```python
from build123d import *

# Parameters (mm, degrees)
BOSS_EXTRUDE1_DEPTH = 25.4
CUT_EXTRUDE1_DEPTH  = 46.597466007


with BuildPart() as part:
    # Sketch1 → Boss-Extrude1 (new body)
    with BuildSketch(Plane.XY):
        Polygon((-31.75, 15.875), (31.75, 15.875), (13.235753401, -19.110856459), (11.70910986, -20.6375), (-11.70910986, -20.6375), (-13.235753401, -19.110856459), align=None)
    extrude(amount=BOSS_EXTRUDE1_DEPTH)

    # Sketch2 → Cut-Extrude1 (cut, through all)
    with BuildSketch(Plane(origin=(0, 0, 0), x_dir=(-1, 0, 0), z_dir=(0, 0, -1))):
        with BuildLine():
            ThreePointArc((-7.4549, -15.76028553), (-9.525, -13.69018553), (-11.5951, -15.76028553))
            ThreePointArc((-11.5951, -15.76028553), (-9.525, -17.83038553), (-7.4549, -15.76028553))
        make_face()
        with BuildLine():
            ThreePointArc((11.5951, -15.76028553), (9.525, -13.69018553), (7.4549, -15.76028553))
            ThreePointArc((7.4549, -15.76028553), (9.525, -17.83038553), (11.5951, -15.76028553))
        make_face()
        with BuildLine():
            ThreePointArc((17.83038553, 9.525), (15.76028553, 11.5951), (13.69018553, 9.525))
            ThreePointArc((13.69018553, 9.525), (15.76028553, 7.4549), (17.83038553, 9.525))
        make_face()
        with BuildLine():
            ThreePointArc((-13.69018553, 9.525), (-15.76028553, 11.5951), (-17.83038553, 9.525))
            ThreePointArc((-17.83038553, 9.525), (-15.76028553, 7.4549), (-13.69018553, 9.525))
        make_face()
        with BuildLine():
            ThreePointArc((-14.2875, 0), (0, -14.2875), (14.2875, 0))
            ThreePointArc((14.2875, 0), (0, 14.2875), (-14.2875, 0))
        make_face()
    extrude(amount=-CUT_EXTRUDE1_DEPTH, mode=Mode.SUBTRACT)


solid = part.part
```
Could you check a few things on this model? Use its own coordinates, in mm. Round coordinates to 2 decimals unless told otherwise and drop trailing zeros. Loops run counter-clockwise (first coordinate to the right, second up) from the corner with the lowest first, then second, coordinate; pieces in that order, holes last. Notation, with made-up numbers: M 68.5,67 L 123.5,67 A36 ccw 123.5,101 Z; hole C -33,20.25 d9. An arc over 180 degrees is marked long. Put each result on its own line as item: value.
Q1. I need wall thicknesses on probe 1 along Y at (x, z) = (0, 8) (1 decimal); probe 2 along Y at (x, z) = (-9, 12.75) (1 decimal); probe 3 along X at (y, z) = (11, 20.75). Which ranges of each line are inside material? Lowest first, please.
Check result:
probe 1: -20.6 to -14.3, 14.3 to 15.9
probe 2: -20.6 to -17.8, -13.8 to -11.1, 11.1 to 15.9
probe 3: -29.17 to -17.21, -14.31 to -9.12, 9.12 to 14.31, 17.21 to 29.17
Q2. Thinking about a two-plate mould opening in Y: for faces 1 (the face through (15, 2, 0)), 2 (the face through (3.097, -13.948, 12.522)), 3 (the face through (-22.363, -1.863, 12.522)), 4 (the face through (0, 15.875, 13)), which applies, released by +Y, released by -Y, zero draft, split by the parting line, or undercut?
Check result:
face 1: zero draft
face 2: undercut
face 3: released by -Y
face 4: released by +Y
Q3. Imagine slicing it at D-D (z = 14.75). State how many separate pieces and enclosed holes the cut face has, then the cut area to 3 significant figures.
Check result:
separate pieces: 1
enclosed holes: 5
area: 917 mm2
Q4. Imagine slicing it at A-A (x = 0). Write out the boundary of the cut face in (y, z) (1 decimal), then the cut area to 3 significant figures.
Check result:
outline: M -20.6,0 L -14.3,0 L -14.3,25.4 L -20.6,25.4 Z; M 14.3,0 L 15.9,0 L 15.9,25.4 L 14.3,25.4 Z
area: 202 mm2
Q5. For pin 1 (3.5 mm diameter, centred on x = -9.52, y = -15.76, fed in from -Z); pin 2 (6 mm diameter, centred on y = -8.5, z = 9, fed in from -X); pin 3 (4 mm diameter, centred on y = -2.5, z = 7.5, fed in from +X); pin 4 (1.5 mm diameter, centred on y = -7, z = 10, fed in from -X), each with a flat end and sliding along its axis, tell me the tip position at first contact or that it passes through.
Check result:
pin 1: through
pin 2: x = -20.44
pin 3: x = 23.08
pin 4: x = -20.04
Q6. Imagine slicing it at C-C (x = 9.5). Write out the boundary of the cut face in (y, z) (1 decimal), then the cut area to 3 significant figures.
Check result:
outline: M -20.6,0 L -17.8,0 L -17.8,25.4 L -20.6,25.4 Z; M -13.7,0 L -10.7,0 L -10.7,25.4 L -13.7,25.4 Z; M 10.7,0 L 15.9,0 L 15.9,25.4 L 10.7,25.4 Z
area: 280 mm2
Q7. Imagine slicing it at B-B (y = 12.5). Write out the boundary of the cut face in (x, z).
Check result:
outline: M -29.96,0 L -6.92,0 L -6.92,25.4 L -29.96,25.4 Z; M 6.92,0 L 29.96,0 L 29.96,25.4 L 6.92,25.4 Z
